Design review of the part built by this model. Coordinates are the model's own, in mm. A direction names the side the tool comes from. Coordinates: 2 decimals unless noted, no trailing zeros. Loops run counter-clockwise (first coordinate to the right, second up) from the corner with the lowest first, then second, coordinate; pieces in that order, holes last. Notation, with made-up numbers: (-28.75, -28) - (-14.75, -28) arc R13 ccw to (-14.75, -23) - close; hole circle Ø4 at (37, -19). An arc over 180 degrees is marked (long way). Answer in a Markdown table with one row per item. Add a question column.
(1) We need section D-D, the plane x = -33. Write out the cut boundary in (y, z), plus the area to 3 significant figures.
(2) To check wall thickness, follow L1, parallel to X at y = 58, z = 6; L2, parallel to Z at x = -24.9, y = 59.6; L3, parallel to Y at x = -24.5, z = 7. State the ranges of each line that lie inside material, in increasing order. Write a range as [from, to].
(3) We need section B-B, the plane x = -24.9. Write out the cut boundary in (y, z).
(4) For faces 5 (the face through (-29.15, 58, 2)), 6 (the face through (-25, 60.72, -1)), 7 (the face through (-15, 72, -12.5)), 8 (the face through (-11.427, 89.38, -12.754)), 9 (the face through (-38.8, 47.3, -12.25)), list the 3-axis set-ups (+Z, -Z, +X, -X, +Y, -Y) from which the entire face can be reached by the end or side of a thin tool; tool diameter is ignored.
(5) The part is to be moulded in two halves that separate along X. For faces 1 (the face through (-43.3, 58, 2)), 2 (the face through (-44.94, 58.18, 7.92)), 3 (the face through (-49.589, 38.778, -12.754)), 4 (the face through (-49, 60.72, 2)), say which applies: released by +X, released by -X, zero draft, split by the parting line, or undercut.
(6) We need section A-A, the plane z = 6.7. Write out the cut boundary in (x, y).
(7) Clearance check with flat-ended pins moving along their axes: pin 1 (3 mm diameter, centred on x = -49, z = 0, fed in from -Y); pin 2 (7.5 mm diameter, centred on x = -48.8, z = 6.7, fed in from -Y); pin 3 (2 mm diameter, centred on x = -22, z = -6, fed in from +Y); pin 4 (1.5 mm diameter, centred on x = -8, y = 90, fed in from -Z). State where each tip first meets the part, or that it passes through.
(8) We need section C-C, the plane z = -10. Write out the cut boundary in (x, y), plus the area to 3 significant figures.
from build123d import *

# Parameters (mm, degrees)
PAD015_DEPTH    = 1
POCKET006_DEPTH = 0.25
CHAMFER003_SIZE = 0.25
POCKET007_DEPTH = 0.25
SKETCH024_W     = 3.05
SKETCH024_H     = 8.1
POCKET008_DEPTH = 0.5
SKETCH025_W     = 8
SKETCH025_H     = 3
PAD016_DEPTH    = 0.5
SKETCH026_W     = 11
SKETCH026_H     = 5
SKETCH026_W_2   = 8.5
PAD017_DEPTH    = 30
SKETCH027_R     = 4.05
SKETCH027_R_2   = 2.75
POCKET009_DEPTH = 54.281
CHAMFER004_SIZE = 1


with BuildPart() as part:
    # Sketch021 (on Face1 of Binder010) → Pad015 (new body)
    with BuildSketch(Plane(origin=(0, 0, -13), x_dir=(1, 0, 0), z_dir=(0, 0, -1))):
        Polygon((4, -110), (-13.313708499, -80.0117772123), (-13.313708499, -47.019624501), (-41.313708499, -47.019624501), (-61, -35.6537388036), (-61, -110), align=None)
    extrude(amount=-PAD015_DEPTH)

    # Sketch022 (on Face8 of Pad015) → Pocket006 (cut)
    with BuildSketch(Plane.XY.offset(-12)):
        Polygon((-13.313708499, 47.019624501), (-41.313708499, 47.019624501), (-61, 35.6537388036), (-61, 36.2310890728), (-41.4476830952, 47.519624501), (-13.313708499, 47.519624501), align=None)
    extrude(amount=-POCKET006_DEPTH, mode=Mode.SUBTRACT)

    # Chamfer003
    chamfer003_edges = [part.edges().sort_by_distance(p)[0] for p in [
        (-61, 73.115545, -12),
        (-28.5, 110, -12),
    ]]
    chamfer(chamfer003_edges, length=CHAMFER003_SIZE)

    # Sketch023 (on Face5 of Chamfer003) → Pocket007 (cut)
    with BuildSketch(Plane.XY.offset(-12)):
        Polygon((-13.313708499, 80.0117772123), (-37.1066017178, 80.0117772123), (-60.75, 103.6551754945), (-60.75, 102.9480687133), (-37.313708499, 79.5117772123), (-13.313708499, 79.5117772123), align=None)
    extrude(amount=-POCKET007_DEPTH, mode=Mode.SUBTRACT)

    # Sketch024 (on Face4 of Pocket007) → Pocket008 (cut)
    with BuildSketch(Plane(origin=(0, 0, -13), x_dir=(1, 0, 0), z_dir=(0, 0, -1))):
        with Locations((-14.838708499, -55.019624501)):
            Rectangle(SKETCH024_W, SKETCH024_H)
        with Locations((-14.838708499, -72.019624501)):
            Rectangle(SKETCH024_W, SKETCH024_H)
        Polygon((-10.838708499, -84.2986029611), (-6.788708499, -91.3134087317), (-9.4300859805, -92.8384087317), (-13.4800859805, -85.8236029611), align=None)
        Polygon((-2.525, -98.6983684806), (1.525, -105.7131742513), (-1.1163774815, -107.2381742513), (-5.1663774815, -100.2233684806), align=None)
    extrude(amount=-POCKET008_DEPTH, mode=Mode.SUBTRACT)

    # Sketch025 (on Face3 of Pocket008) → Pad016 (join)
    with BuildSketch(Plane(origin=(0, 0, -13), x_dir=(1, 0, 0), z_dir=(0, 0, -1))):
        with Locations((-27.713708499, -45.519624501)):
            Rectangle(SKETCH025_W, SKETCH025_H)
        Polygon((-47.5766062413, -43.4037388036), (-54.5048094716, -39.4037388036), (-53.0048094716, -36.8056625922), (-46.0766062413, -40.8056625922), align=None)
    extrude(amount=-PAD016_DEPTH)

    # Sketch026 (on Face28 of Pad016) → Pad017 (join)
    with BuildSketch(Plane.XY.offset(-12)):
        with Locations((-48.8, 58.22)):
            Rectangle(SKETCH026_W, SKETCH026_H)
        with Locations((-24.9, 58.22)):
            Rectangle(SKETCH026_W_2, SKETCH026_H)
    extrude(amount=PAD017_DEPTH)

    # Sketch027 (on Face45 of Pad017) → Pocket009 (cut, through all)
    with BuildSketch(Plane.XZ.offset(-55.72)):
        with Locations((-48.8, 6.7)):
            Circle(SKETCH027_R)
        with Locations((-24.9, 13.15)):
            Circle(SKETCH027_R_2)
    extrude(amount=-POCKET009_DEPTH, mode=Mode.SUBTRACT)

    # Chamfer004
    chamfer004_edges = [part.edges().sort_by_distance(p)[0] for p in [
        (-54.3, 60.72, 3),
        (-54.3, 58.22, 18),
        (-48.8, 60.72, 18),
        (-43.3, 58.22, 18),
        (-48.8, 55.72, 18),
        (-54.3, 55.72, 3),
        (-43.3, 55.72, 3),
        (-29.15, 60.72, 3),
        (-29.15, 58.22, 18),
        (-24.9, 60.72, 18),
        (-24.9, 55.72, 18),
        (-29.15, 55.72, 3),
        (-43.3, 60.72, 3),
        (-20.65, 55.72, 3),
        (-20.65, 60.72, 3),
        (-20.65, 58.22, 18),
    ]]
    chamfer(chamfer004_edges, length=CHAMFER004_SIZE)


solid = part.part
Responses:
| question | item | result |
|---|---|---|
| 1 | outline | (47.02, -13) - (110, -13) - (110, -12.25) - (109.75, -12) - (80.01, -12) - (80.01, -12.25) - (79.51, -12.25) - (79.51, -12) - (47.52, -12) - (47.52, -12.25) - (47.02, -12.25) - close |
| 1 | area | 62.7 mm2 |
| 2 | L1 | x = [-54.3, -52.79], [-44.81, -43.3], [-29.15, -20.65] |
| 2 | L2 | z = [-13, 10.4], [15.9, 18] |
| 2 | L3 | y = [55.72, 60.72] |
| 3 | outline | (44.02, -13) - (110, -13) - (110, -12.25) - (109.75, -12) - (80.01, -12) - (80.01, -12.25) - (79.51, -12.25) - (79.51, -12) - (60.72, -12) - (60.72, 10.4) - (55.72, 10.4) - (55.72, -12) - (47.52, -12) - (47.52, -12.25) - (47.02, -12.25) - (47.02, -12.5) - (44.02, -12.5) - close; (55.72, 15.9) - (60.72, 15.9) - (60.72, 17) - (59.72, 18) - (56.72, 18) - (55.72, 17) - close |
| 4 | face 5 | +Z, +Y, -Y |
| 4 | face 6 | +Z, +X, -X, +Y |
| 4 | face 7 | -Z, +X |
| 4 | face 8 | -Z |
| 4 | face 9 | +Z, +X, -Y |
| 5 | face 1 | undercut |
| 5 | face 2 | undercut |
| 5 | face 3 | released by +X |
| 5 | face 4 | zero draft |
| 6 | outline | (-54.3, 56.72) - (-53.3, 55.72) - (-52.85, 55.72) - (-52.85, 60.72) - (-53.3, 60.72) - (-54.3, 59.72) - close; (-44.75, 55.72) - (-44.3, 55.72) - (-43.3, 56.72) - (-43.3, 59.72) - (-44.3, 60.72) - (-44.75, 60.72) - close; (-29.15, 56.72) - (-28.15, 55.72) - (-21.65, 55.72) - (-20.65, 56.72) - (-20.65, 59.72) - (-21.65, 60.72) - (-28.15, 60.72) - (-29.15, 59.72) - close |
| 7 | pin 1 | stops at y = 55.72 |
| 7 | pin 2 | passes through |
| 7 | pin 3 | stops at y = 60.72 |
| 7 | pin 4 | stops at z = -12.5 |
| 8 | outline | (-54.3, 56.72) - (-53.3, 55.72) - (-44.3, 55.72) - (-43.3, 56.72) - (-43.3, 59.72) - (-44.3, 60.72) - (-53.3, 60.72) - (-54.3, 59.72) - close; (-29.15, 56.72) - (-28.15, 55.72) - (-21.65, 55.72) - (-20.65, 56.72) - (-20.65, 59.72) - (-21.65, 60.72) - (-28.15, 60.72) - (-29.15, 59.72) - close |
| 8 | area | 93.5 mm2 |
